```python
from build123d import *

# Parameters (mm, degrees)
CHANFREIN1_SIZE = 0.5


with BuildPart() as part:
    # Esquisse1 → Révolution1 (revolve)
    with BuildSketch(Plane.XY):
        Polygon((0, 0), (0, 2.5), (6.5, 2.5), (6.5, 3), (14.5, 3), (14.5, 2.5), (21, 2.5), (21, 0), align=None)
    revolve(axis=Axis((-54.824636662, 0, 0), (1, 0, 0)))

    # Chanfrein1
    chanfrein1_edges = [part.edges().sort_by_distance(p)[0] for p in [
        (21, -2.5, 0),
        (0, -2.5, 0),
    ]]
    chamfer(chanfrein1_edges, length=CHANFREIN1_SIZE)


solid = part.part
```
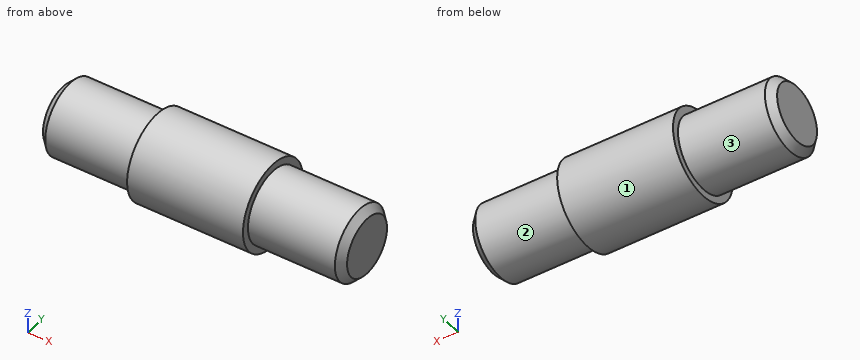
Design review of the part built by this model. Coordinates are the model's own, in mm. Face numbers are marked on the shaded views. A direction names the side the tool comes from. Round coordinates to 2 decimals unless told otherwise and drop trailing zeros. Write each loop counter-clockwise with the first axis right and the second up, starting at its lowest first coordinate (ties: lowest second). Pieces come first, ordered by that corner, then holes.
Item 1: We need section C-C on x = 7.5. Write out the cut boundary in (y, z).
Item 2: For probe 1 along X at (y, z) = (-2.65, 0.1); probe 2 along Y at (x, z) = (13.5, 0.1); probe 3 along Z at (x, y) = (17, 0.15), list the stretches that pass through material, from the lowest coordinate up.
Item 3: For the marked faces 1, 2 and 3, list the 3-axis set-ups (+Z, -Z, +X, -X, +Y, -Y) from which the entire face can be reached by the end or side of a thin tool; tool diameter is ignored.
Item 4: We need section D-D on x = 17.75. Write out the cut boundary in (y, z).
Item 5: We need section A-A on z = 0. Write out the cut boundary in (x, y).
Item 6: Clearance check with a flat-ended pin moving along its axis: pin 1 Ø2 at (x, y) = (17, -1.5) entering from -Z. State where the tip first meets the part, or that it passes through.
Returned:
1. outline: circle Ø6 at (0, 0)
2. probe 1: x = 6.5 to 14.5
2. probe 2: y = -3 to 3
2. probe 3: z = -2.5 to 2.5
3. face 1: +X, -X
3. face 2: +X
3. face 3: -X
4. outline: circle Ø5 at (0, 0)
5. outline: (0, -2) - (0.5, -2.5) - (6.5, -2.5) - (6.5, -3) - (14.5, -3) - (14.5, -2.5) - (20.5, -2.5) - (21, -2) - (21, 2) - (20.5, 2.5) - (14.5, 2.5) - (14.5, 3) - (6.5, 3) - (6.5, 2.5) - (0.5, 2.5) - (0, 2) - close
6. pin 1: stops at z = -2.45
